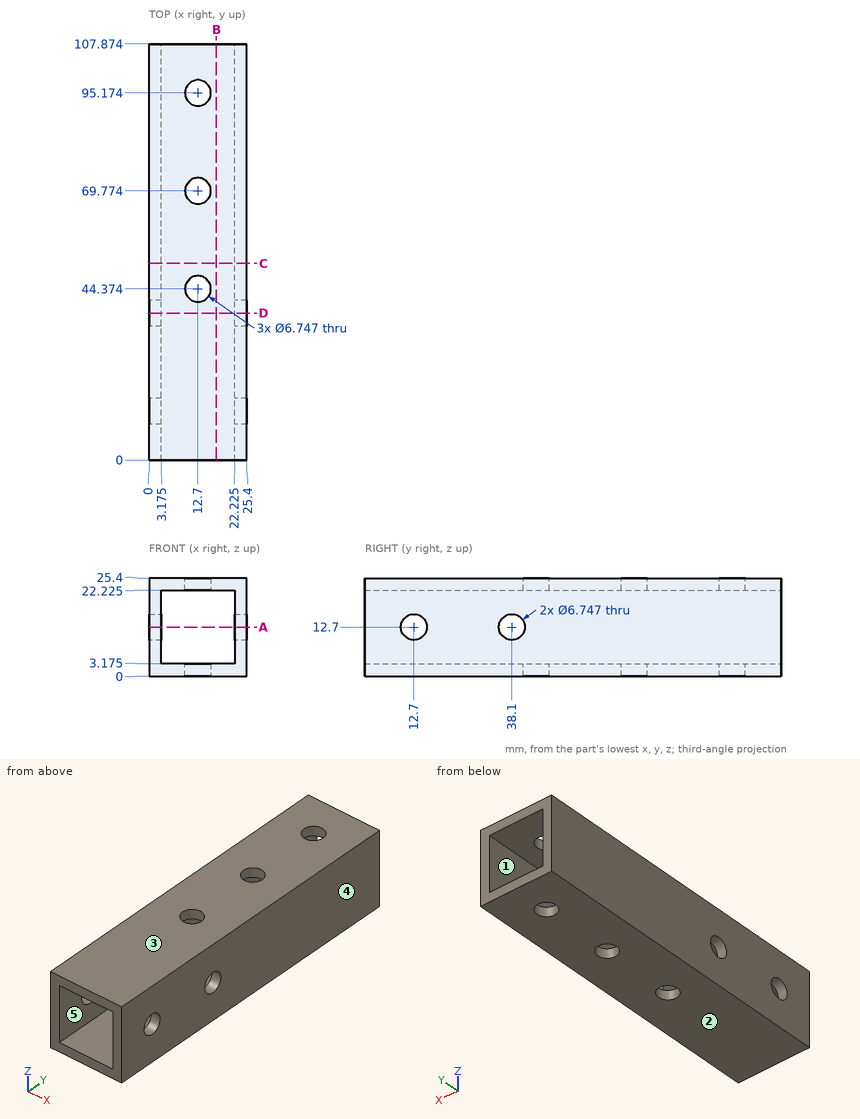
The figure shows three views and two pictorial views of one solid part (mm, origin at its lowest corner). Answer the questions. A direction names the side the tool comes from. Give positions to 0.01 mm unless a question says otherwise; leave off trailing zeros. Write each loop counter-clockwise with the first axis right and the second up, starting at its lowest first coordinate (ties: lowest second). Pieces come first, ordered by that corner, then holes. Notation, with made-up numbers: (8, 64) - (23, 64) arc R15 ccw to (23, 77) - close; hole circle Ø8 at (-6.5, 40.5). An arc over 180 degrees is marked (long way). Use one line per item in the form item = value. Start each with the question number.
1) Find section A-A on z = 12.7. Determine the outline of the cut face in (x, y) (1 decimal), plus the area to 3 significant figures.
2) A tool of negligible diameter and unlimited length cuts with its end or side. For the marked faces 1 and 2, from which of +Z, -Z, +X, -X, +Y, -Y can it reach the whole face along a straight path? Write none if from no direction.
3) Find section D-D on y = 38.1. Determine the outline of the cut face in (x, z) (1 decimal).
4) Consider line 1 along Y through (x, z) = (12.7, 23.2); line 2 along Y through (x, z) = (0.7, 12.7); line 3 along X through (y, z) = (32, 9.5) (3 decimals). Determine where each line is inside the solid, lowest interval first. Write a range as from..to.
5) A flat-ended cylindrical pin translates along its axis: pin 1 Ø6 at (x, y) = (12.7, 69.77) entering from -Z. Find the tip coordinate at first contact, or state that the pin passes through.
6) Find section C-C on y = 51. Determine the outline of the cut face in (x, z) (3 decimals).
7) The mould has two halves that part along X. Classify the marked faces 3, 4 and 5: pulls with the +X half, pulls with the -X half, needs draft (parallel to the pull), parting line crosses it, or undercut.
8) Find section B-B on x = 17.5. Determine the outline of the cut face in (y, z) (1 decimal), plus the area to 3 significant figures.
Geometry results:
q1.outline = (0, 0) - (3.2, 0) - (3.2, 9.3) - (0, 9.3) - close; (0, 16.1) - (3.2, 16.1) - (3.2, 34.7) - (0, 34.7) - close; (0, 41.5) - (3.2, 41.5) - (3.2, 107.9) - (0, 107.9) - close; (22.2, 0) - (25.4, 0) - (25.4, 9.3) - (22.2, 9.3) - close; (22.2, 16.1) - (25.4, 16.1) - (25.4, 34.7) - (22.2, 34.7) - close; (22.2, 41.5) - (25.4, 41.5) - (25.4, 107.9) - (22.2, 107.9) - close
q1.area = 599 mm2
q2.face_1 = +Y, -Y
q2.face_2 = -Z, +X, -X, +Y, -Y
q3.outline = (0, 0) - (25.4, 0) - (25.4, 9.3) - (22.2, 9.3) - (22.2, 3.2) - (3.2, 3.2) - (3.2, 9.3) - (0, 9.3) - close; (0, 16.1) - (3.2, 16.1) - (3.2, 22.2) - (22.2, 22.2) - (22.2, 16.1) - (25.4, 16.1) - (25.4, 25.4) - (0, 25.4) - close
q4.line_1 = 0..41, 47.75..66.4, 73.15..91.8, 98.55..107.87
q4.line_2 = 0..9.33, 16.07..34.73, 41.47..107.87
q4.line_3 = 0..3.175, 22.225..25.4
q5.pin_1 = through
q6.outline = (0, 0) - (25.4, 0) - (25.4, 25.4) - (0, 25.4) - close; hole (3.175, 3.175) - (22.225, 3.175) - (22.225, 22.225) - (3.175, 22.225) - close
q7.face_3 = needs draft
q7.face_4 = pulls with the +X half
q7.face_5 = undercut
q8.outline = (0, 0) - (107.9, 0) - (107.9, 3.2) - (0, 3.2) - close; (0, 22.2) - (107.9, 22.2) - (107.9, 25.4) - (0, 25.4) - close
q8.area = 685 mm2
